```python
from build123d import *

# Parameters (mm, degrees)
SKETCH1_W                       = 165.1
SKETCH1_H                       = 12.7
BOSS_EXTRUDE1_DEPTH             = 128.5875
SKETCH2_R                       = 20.6375
CUT_EXTRUDE1_DEPTH              = 154.33146336
CUT_EXTRUDE3_DEPTH              = 154.33146336
FILLET1_R                       = 3.175
FILLET2_R                       = 1.5875
SKETCH5_W                       = 101.6
SKETCH5_H                       = 9.525
CUT_EXTRUDE4_DEPTH              = 154.33146336
FILLET3_R                       = 3.175
F_21_0_159_DIAMETER_HOLE2_D     = 4.0386
F_21_0_159_DIAMETER_HOLE2_DEPTH = 20.6375
F_21_0_159_DIAMETER_HOLE2_TIP   = 1.213317848
CUT_EXTRUDE5_DEPTH              = 154.33146336


# Read off the part's stored shape, not the designer's step: #21 (0.159) Diameter Hole1
with BuildPart() as part:
    # Sketch1 → Boss-Extrude1 (new, symmetric)
    with BuildSketch(Plane(origin=(0, 0, 0), x_dir=(1, 0, 0), z_dir=(0, 1, 0))):
        Rectangle(SKETCH1_W, SKETCH1_H)
    extrude(amount=BOSS_EXTRUDE1_DEPTH, both=True)

    # Sketch2 → Cut-Extrude1 (cut, through all)
    with BuildSketch(Plane.XY.offset(6.35)):
        with Locations((0, 128.5875)):
            Circle(SKETCH2_R)
    extrude(amount=-CUT_EXTRUDE1_DEPTH, mode=Mode.SUBTRACT)

    # Sketch4 → Cut-Extrude3 (cut, through all)
    with BuildSketch(Plane.XY.offset(6.35)):
        with BuildLine():
            Line((57.277, 128.5875), (57.277, 106.3625))
            Line((57.277, 106.3625), (43.877983689, 106.3625))
            Line((43.877983689, 106.3625), (38.415384653, 115.823999072))
            ThreePointArc((38.415384653, 115.823999072), (39.623999536, 120.334615615), (44.134615883, 119.126))
            Line((44.134615883, 119.126), (47.690804866, 112.9665))
            Line((47.690804866, 112.9665), (50.673, 112.9665))
            Line((50.673, 112.9665), (50.673, 128.5875))
            Line((50.673, 128.5875), (57.277, 128.5875))
        make_face()
        with BuildLine():
            Line((-50.673, 128.5875), (-57.277, 128.5875))
            Line((-57.277, 128.5875), (-57.277, 106.3625))
            Line((-57.277, 106.3625), (-43.877983689, 106.3625))
            Line((-43.877983689, 106.3625), (-38.415384653, 115.823999072))
            ThreePointArc((-38.415384653, 115.823999072), (-39.623999536, 120.334615615), (-44.134615883, 119.126))
            Line((-44.134615883, 119.126), (-47.690804866, 112.9665))
            Line((-47.690804866, 112.9665), (-50.673, 112.9665))
            Line((-50.673, 112.9665), (-50.673, 128.5875))
        make_face()
    extrude(amount=-CUT_EXTRUDE3_DEPTH, mode=Mode.SUBTRACT)

    # Fillet1
    fillet1_edges = [part.edges().sort_by_distance(p)[0] for p in [
        (50.673, 128.5875, 0),
        (57.277, 128.5875, 0),
        (57.277, 106.3625, 0),
        (43.877983689, 106.3625, 0),
        (-43.877983689, 106.3625, 0),
        (-57.277, 106.3625, 0),
        (-57.277, 128.5875, 0),
        (-50.673, 128.5875, 0),
    ]]
    fillet(fillet1_edges, radius=FILLET1_R)

    # Fillet2
    fillet2_edges = [part.edges().sort_by_distance(p)[0] for p in [
        (47.690804866, 112.9665, 0),
        (50.673, 112.9665, 0),
        (-50.673, 112.9665, 0),
        (-47.690804866, 112.9665, 0),
    ]]
    fillet(fillet2_edges, radius=FILLET2_R)

    # Sketch5 → Cut-Extrude4 (cut, through all)
    with BuildSketch(Plane.XY.offset(6.35)):
        with Locations((0, -123.825)):
            Rectangle(SKETCH5_W, SKETCH5_H)
    extrude(amount=-CUT_EXTRUDE4_DEPTH, mode=Mode.SUBTRACT)

    # Fillet3
    fillet3_edges = [part.edges().sort_by_distance(p)[0] for p in [
        (-50.8, -128.5875, 0),
        (-50.8, -119.0625, 0),
        (50.8, -119.0625, 0),
        (50.8, -128.5875, 0),
    ]]
    fillet(fillet3_edges, radius=FILLET3_R)

    # #21 (0.159) Diameter Hole1 outline → #21 (0.159) Diameter Hole1 (revolve, cut)
    with BuildSketch(Plane(origin=(0, 111.412500004, 0), x_dir=(0, 1, 0), z_dir=(0, 0, -1))):
        Polygon((0, 82.55), (0, 60.699182152), (2.0193, 61.9125), (2.0193, 82.55), align=None)
    revolve(axis=Axis((0, 111.412500004, 0), (1, 0, 0)), mode=Mode.SUBTRACT)

    # 21 _0.159_ Diameter Hole1 2 outline → 21 _0.159_ Diameter Hole1 2 (revolve, cut)
    with BuildSketch(Plane(origin=(0, 79.412500004, 0), x_dir=(0, 1, 0), z_dir=(0, 0, -1))):
        Polygon((0, 82.55), (0, 60.699182152), (2.0193, 61.9125), (2.0193, 82.55), align=None)
    revolve(axis=Axis((0, 79.412500004, 0), (1, 0, 0)), mode=Mode.SUBTRACT)

    # 21 _0.159_ Diameter Hole1 3 outline → 21 _0.159_ Diameter Hole1 3 (revolve, cut)
    with BuildSketch(Plane(origin=(0, 15.412500004, 0), x_dir=(0, 1, 0), z_dir=(0, 0, -1))):
        Polygon((0, 82.55), (0, 60.699182152), (2.0193, 61.9125), (2.0193, 82.55), align=None)
    revolve(axis=Axis((0, 15.412500004, 0), (1, 0, 0)), mode=Mode.SUBTRACT)

    # 21 _0.159_ Diameter Hole1 4 outline → 21 _0.159_ Diameter Hole1 4 (revolve, cut)
    with BuildSketch(Plane(origin=(0, -16.587499996, 0), x_dir=(0, 1, 0), z_dir=(0, 0, -1))):
        Polygon((0, 82.55), (0, 60.699182152), (2.0193, 61.9125), (2.0193, 82.55), align=None)
    revolve(axis=Axis((0, -16.587499996, 0), (1, 0, 0)), mode=Mode.SUBTRACT)

    # 21 _0.159_ Diameter Hole1 5 outline → 21 _0.159_ Diameter Hole1 5 (revolve, cut)
    with BuildSketch(Plane(origin=(0, -80.587499996, 0), x_dir=(0, 1, 0), z_dir=(0, 0, -1))):
        Polygon((0, 82.55), (0, 60.699182152), (2.0193, 61.9125), (2.0193, 82.55), align=None)
    revolve(axis=Axis((0, -80.587499996, 0), (1, 0, 0)), mode=Mode.SUBTRACT)

    # 21 _0.159_ Diameter Hole1 6 outline → 21 _0.159_ Diameter Hole1 6 (revolve, cut)
    with BuildSketch(Plane(origin=(0, -112.587499996, 0), x_dir=(0, 1, 0), z_dir=(0, 0, -1))):
        Polygon((0, 82.55), (0, 60.699182152), (2.0193, 61.9125), (2.0193, 82.55), align=None)
    revolve(axis=Axis((0, -112.587499996, 0), (1, 0, 0)), mode=Mode.SUBTRACT)

    # #21 (0.159) Diameter Hole2
    with Locations(Plane.ZY.offset(82.55)):
        with Locations((0, -112.587499996), (0, -80.587499996), (0, -16.587499996), (0, 15.412500004), (0, 79.412500004), (0, 111.412500004)):
            Hole(F_21_0_159_DIAMETER_HOLE2_D / 2, depth=F_21_0_159_DIAMETER_HOLE2_DEPTH)
            with Locations((0, 0, -(F_21_0_159_DIAMETER_HOLE2_DEPTH + F_21_0_159_DIAMETER_HOLE2_TIP / 2))):  # 118° drill point
                Cone(0, F_21_0_159_DIAMETER_HOLE2_D / 2, F_21_0_159_DIAMETER_HOLE2_TIP, mode=Mode.SUBTRACT)

    # Sketch10 → Cut-Extrude5 (cut, through all)
    with BuildSketch(Plane.XY.offset(6.35)):
        with BuildLine():
            Line((-60.30687725, -90.072420775), (-49.195816982, 36.927579225))
            ThreePointArc((-49.195816982, 36.927579225), (-44.036360507, 41.25687725), (-39.707062483, 36.097420775))
            Line((-39.707062483, 36.097420775), (-50.81812275, -90.902579225))
            ThreePointArc((-50.81812275, -90.902579225), (-55.977579225, -95.23187725), (-60.30687725, -90.072420775))
        make_face()
        with BuildLine():
            Line((-25.41812275, -90.902579225), (-14.307062483, 36.097420775))
            ThreePointArc((-14.307062483, 36.097420775), (-18.636360507, 41.25687725), (-23.795816982, 36.927579225))
            Line((-23.795816982, 36.927579225), (-34.90687725, -90.072420775))
            ThreePointArc((-34.90687725, -90.072420775), (-30.577579225, -95.23187725), (-25.41812275, -90.902579225))
        make_face()
        with BuildLine():
            Line((-0.01812275, -90.902579225), (11.092937517, 36.097420775))
            ThreePointArc((11.092937517, 36.097420775), (6.763639493, 41.25687725), (1.604183018, 36.927579225))
            Line((1.604183018, 36.927579225), (-9.50687725, -90.072420775))
            ThreePointArc((-9.50687725, -90.072420775), (-5.177579225, -95.23187725), (-0.01812275, -90.902579225))
        make_face()
        with BuildLine():
            Line((25.38187725, -90.902579225), (36.492937517, 36.097420775))
            ThreePointArc((36.492937517, 36.097420775), (32.163639493, 41.25687725), (27.004183018, 36.927579225))
            Line((27.004183018, 36.927579225), (15.89312275, -90.072420775))
            ThreePointArc((15.89312275, -90.072420775), (20.222420775, -95.23187725), (25.38187725, -90.902579225))
        make_face()
        with BuildLine():
            Line((50.78187725, -90.902579225), (61.892937517, 36.097420775))
            ThreePointArc((61.892937517, 36.097420775), (57.563639493, 41.25687725), (52.404183018, 36.927579225))
            Line((52.404183018, 36.927579225), (41.29312275, -90.072420775))
            ThreePointArc((41.29312275, -90.072420775), (45.622420775, -95.23187725), (50.78187725, -90.902579225))
        make_face()
    extrude(amount=-CUT_EXTRUDE5_DEPTH, mode=Mode.SUBTRACT)


solid = part.part
```
Part model, mm, in its own coordinate system. A direction names the side the tool comes from. Round coordinates to 2 decimals unless told otherwise and drop trailing zeros. Write each loop counter-clockwise with the first axis right and the second up, starting at its lowest first coordinate (ties: lowest second). Pieces come first, ordered by that corner, then holes.
Item 1: Drop flat-ended pins along their axis: pin 1 Ø2.5 at (y, z) = (15.41, 0) entering from +X; pin 2 Ø4 at (x, z) = (33.5, 4.5) entering from -Y; pin 3 Ø3.5 at (y, z) = (-80.59, 0) entering from -X; pin 4 Ø3 at (x, y) = (3.5, 36) entering from +Z. Give the stop position or say it passes through.
Results:
pin 1: stops at x = 61.45
pin 2: stops at y = -119.06
pin 3: stops at x = -61.75
pin 4: passes through
Item 2: Cut at C-C, the plane z = 4. Count the separate pieces of the cut face and the enclosed holes in it, plus the area to 3 significant figures.
Results:
separate pieces: 1
enclosed holes: 5
area: 33,900 mm2
Item 3: Cut at B-B, the plane x = 67.5. Give the cut face in (y, z), plus the area to 3 significant figures.
Results:
outline: (-128.59, -6.35) - (128.59, -6.35) - (128.59, 6.35) - (-128.59, 6.35) - close; hole circle Ø4.04 at (-112.59, 0); hole circle Ø4.04 at (-80.59, 0); hole circle Ø4.04 at (-16.59, 0); hole circle Ø4.04 at (15.41, 0); hole circle Ø4.04 at (79.41, 0); hole circle Ø4.04 at (111.41, 0)
area: 3,190 mm2
Item 4: Probe L1, parallel to X at y = -91, z = 3.25; L2, parallel to X at y = 111.5, z = 4; L3, parallel to X at y = -86, z = 5. List the from-to ranges inside material, lowest first.
Results:
L1: x = -82.55 to -60.3, -50.83 to -34.9, -25.43 to -9.5, -0.03 to 15.9, 25.37 to 41.3, 50.77 to 82.55
L2: x = -82.55 to -57.28, -40.91 to -11.57, 11.57 to 40.91, 57.28 to 82.55
L3: x = -82.55 to -59.95, -50.39 to -34.55, -24.99 to -9.15, 0.41 to 16.25, 25.81 to 41.65, 51.21 to 82.55
Item 5: Which spindle directions (+Z, -Z, +X, -X, +Y, -Y) get a long thin tool onto all of the face, cutting with end or side? Do faces 1 (the flat face through (21.526, -25.683, 0.089)), 2 (the flat face through (-57.277, 118, 0)), 3 (the flat face through (-1, -119.062, 0)). Say none if no direction does.
Results:
face 1: +Z, -Z
face 2: +Z, -Z, +Y
face 3: +Z, -Z, -Y
Item 6: Two-plate mould, pull along X, no slides. Class faces 4 (the cylindrical face through (-30.68, -95.22, 0.09)), 5 (the flat face through (82.55, 2, 0)), 6 (the flat face through (71, 128.588, 0)): +X half, -X half, draft (parallel to the pull), parting line (faces both ways), or undercut.
Results:
face 4: undercut
face 5: +X half
face 6: draft
Item 7: Cut at A-A, the plane y = -23. Give the cut face in (x, z).
Results:
outline: (-82.55, -6.35) - (-54.44, -6.35) - (-54.44, 6.35) - (-82.55, 6.35) - close; (-44.88, -6.35) - (-29.04, -6.35) - (-29.04, 6.35) - (-44.88, 6.35) - close; (-19.48, -6.35) - (-3.64, -6.35) - (-3.64, 6.35) - (-19.48, 6.35) - close; (5.92, -6.35) - (21.76, -6.35) - (21.76, 6.35) - (5.92, 6.35) - close; (31.32, -6.35) - (47.16, -6.35) - (47.16, 6.35) - (31.32, 6.35) - close; (56.72, -6.35) - (82.55, -6.35) - (82.55, 6.35) - (56.72, 6.35) - close
